For this review, take the finished solid that the model builds, in its own axes (mm). Face numbers are marked on the shaded views. Give positions to 0.01 mm unless a question says otherwise; leave off trailing zeros. Loops run counter-clockwise (first coordinate to the right, second up) from the corner with the lowest first, then second, coordinate; pieces in that order, holes last.
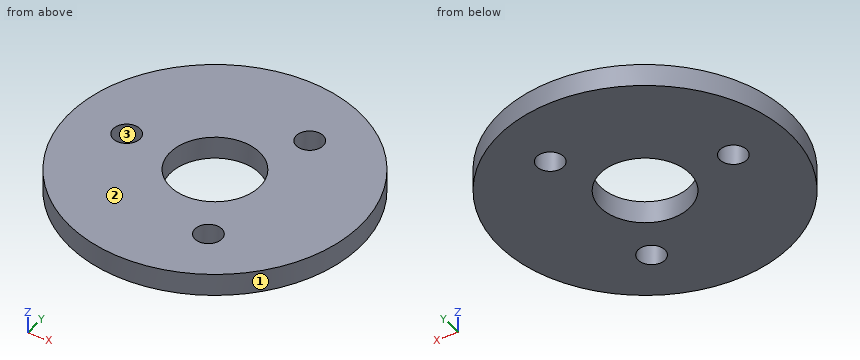
```python
from build123d import *

# Parameters (mm, degrees)
SKETCH1_R           = 32.5
SKETCH1_R_2         = 10
SKETCH1_R_3         = 3
BOSS_EXTRUDE1_DEPTH = 2.5


with BuildPart() as part:
    # Sketch1 → Boss-Extrude1 (new, symmetric)
    with BuildSketch(Plane(origin=(0, 0, 0), x_dir=(0, 1, 0), z_dir=(0, 0, 1))):
        with Locations(Location((0, 0, 0), (0, 0, 270))):
            Circle(SKETCH1_R)
        with Locations(Location((0, 0, 0), (0, 0, 270))):
            Circle(SKETCH1_R_2, mode=Mode.SUBTRACT)
        with Locations(Location((0, 20, 0), (0, 0, 270))):
            Circle(SKETCH1_R_3, mode=Mode.SUBTRACT)
        with Locations(Location((17.320508076, -10, 0), (0, 0, 270))):
            Circle(SKETCH1_R_3, mode=Mode.SUBTRACT)
        with Locations(Location((-17.320508076, -10, 0), (0, 0, 270))):
            Circle(SKETCH1_R_3, mode=Mode.SUBTRACT)
    extrude(amount=BOSS_EXTRUDE1_DEPTH, both=True)


solid = part.part
```
Q1. For probe 1 along Y at (x, z) = (0, -1.2); probe 2 along Y at (x, z) = (7.5, -0.3); probe 3 along Y at (x, z) = (10.5, -1.15), list the stretches that pass through material, from the lowest coordinate up.
Answers:
probe 1: y = -32.5 to -10, 10 to 32.5
probe 2: y = -31.62 to -18.98, -15.66 to -6.61, 6.61 to 15.66, 18.98 to 31.62
probe 3: y = -30.76 to -20.28, -14.36 to 14.36, 20.28 to 30.76
Q2. Consider section B-B on x = 0. Give the boundary of the cut face in (y, z).
Answers:
outline: (-32.5, -2.5) - (-10, -2.5) - (-10, 2.5) - (-32.5, 2.5) - close; (10, -2.5) - (32.5, -2.5) - (32.5, 2.5) - (10, 2.5) - close
Q3. Mouldability with a two-part tool opening along Y and no side actions: class the marked faces 1, 2 and 3 as +Y half, -Y half, draft (parallel to the pull), parting line (faces both ways), or undercut.
Answers:
face 1: parting line
face 2: draft
face 3: undercut
Q4. For pin 1 Ø5 at (x, y) = (-20, 0) entering from -Z; pin 2 Ø1 at (y, z) = (20, -1.5) entering from +X; pin 3 Ø1 at (y, z) = (-15, 0) entering from +X; pin 4 Ø1 at (y, z) = (11.5, 2) entering from +X, all flat-tipped, find the tip position at first contact; note any pin that passes through.
Answers:
pin 1: passes through
pin 2: stops at x = 26
pin 3: stops at x = 29.09
pin 4: stops at x = 30.58
Q5. Consider section A-A on y = 0. Give the boundary of the cut face in (x, z).
Answers:
outline: (-32.5, -2.5) - (-23, -2.5) - (-23, 2.5) - (-32.5, 2.5) - close; (-17, -2.5) - (-10, -2.5) - (-10, 2.5) - (-17, 2.5) - close; (10, -2.5) - (32.5, -2.5) - (32.5, 2.5) - (10, 2.5) - close
Q6. Consider section D-D on z = -0.85. Give the boundary of the cut face in (x, y), plus the area to 3 significant figures.
Answers:
outline: circle Ø65 at (0, 0); hole circle Ø6 at (-20, 0); hole circle Ø20 at (0, 0); hole circle Ø6 at (10, -17.32); hole circle Ø6 at (10, 17.32)
area: 2,920 mm2
Q7. Consider section C-C on y = 8. Give the boundary of the cut face in (x, z).
Answers:
outline: (-31.5, -2.5) - (-6, -2.5) - (-6, 2.5) - (-31.5, 2.5) - close; (6, -2.5) - (31.5, -2.5) - (31.5, 2.5) - (6, 2.5) - close
